Here's how the part is built. I have some questions about the finished solid (model axes, mm). Face numbers are marked on the shaded views. A direction names the side the tool comes from. Round coordinates to 2 decimals unless told otherwise and drop trailing zeros. Loops run counter-clockwise (first coordinate to the right, second up) from the corner with the lowest first, then second, coordinate; pieces in that order, holes last. Notation, with made-up numbers: (31.5, 59.5) -> (57.5, 59.5) arc R22 cw to (57.5, 72.5) -> close; hole circle Ø3 at (48.25, 22). An arc over 180 degrees is marked (long way). One line per item, written item: value. Start each with the question number.
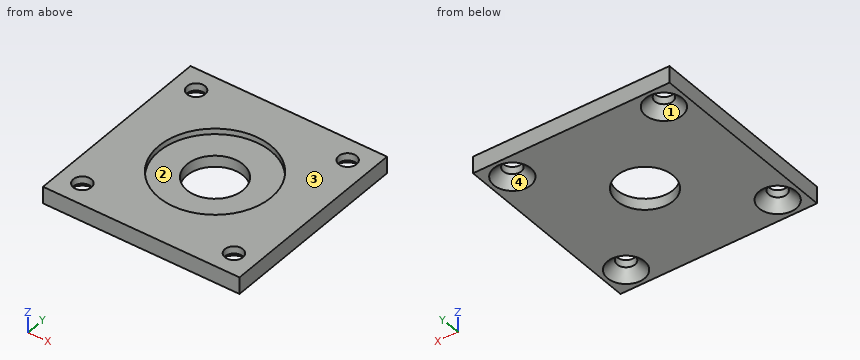
Autodesk Inventor part; units mm, degrees
ref_plane "YZ Plane" through (0, 0, 0) normal (1, 0, 0) x (0, 1, 0)
ref_plane "XZ Plane" through (0, 0, 0) normal (0, 1, 0) x (-1, 0, 0)
ref_plane "XY Plane" through (0, 0, 0) normal (0, 0, 1) x (1, 0, 0)
sketch "Sketch1" plane through (0, 0, 0) normal (0, 0, 1) x (1, 0, 0)
  line L0 (17.5, -17.5) -> (-17.5, -17.5)
  line L1 (-17.5, -17.5) -> (-17.5, 17.5)
  line L2 (-17.5, 17.5) -> (17.5, 17.5)
  line L3 (17.5, 17.5) -> (17.5, -17.5)
  line L4 (17.5, -17.5) -> (-17.5, 17.5) construction
  line L5 (-17.5, -17.5) -> (17.5, 17.5) construction
  circle A0 centre (-13.4987, -13.4987) radius 1.5
  circle A1 centre (13.4987, -13.4987) radius 1.5
  circle A2 centre (13.4987, 13.4987) radius 1.5
  circle A3 centre (-13.4987, 13.4987) radius 1.5
  circle A4 centre (0, 0) radius 5
  circle A5 centre (0, 0) radius 10
  dimension "d0" = 35
  dimension "d1" = 35
  dimension "d3" = 3
  dimension "d6" = 360
  dimension "d8" = 10
  dimension "d9" = 20
extrude "Extrusion1" add sketch "Sketch1" against normal blind 3 contours L0 L1 L2 L3 | A0 | A1 | A2 | A3 | A5
extrude "Extrusion2" cut sketch "Sketch1" against normal blind 1 contours A5
sketch "Sketch2" plane through (0, 0, -3) normal (0, 0, -1) x (-1, 0, 0)
  circle A0 centre (13.4987, 13.4987) radius 1.5
  circle A1 centre (-13.4987, 13.4987) radius 1.5
  circle A2 centre (-13.4987, -13.4987) radius 1.5
  circle A3 centre (13.4987, -13.4987) radius 1.5
  point P0 (0, 0)
hole "Hole2" at (13.4987, 13.4987, -3) at (-13.4987, 13.4987, -3) at (-13.4987, -13.4987, -3) at (13.4987, -13.4987, -3) direction (0, 0, 1) diameter 3.2 depth 3 countersink diameter 6.6 countersink angle 90
properties part number "АНЦП.014.00.00.004" material "PET Plastic"
Q1. Which directions (+Z, -Z, +X, -X, +Y, -Y) give clear straight access to the entire face, cutting with the end or side of a thin tool? Please do the marked faces 1 and 2.
Q2. If we mould it in two halves opening along Y, with no side actions, what happens to the marked faces 3 and 4? For each: released by +Y, released by -Y, zero draft, split by the parting line, or undercut.
Q3. If I drill on line 1 along Y through (x, z) = (-12, -1.9); line 2 along Y through (x, z) = (0, -2.15); line 3 along Y through (x, z) = (-13, -1.45), over which ranges is the centre line in solid material (lowest first)?
Q4. I want a section at D-D on x = -6. Please give me the cut outline in (y, z).
Q5. Will these pins go through, and if not, where does the flat tip stop? P1, Ø12, axis at x = 0, y = 0, coming from the +Z side; P2, Ø5, axis at x = 13.5, y = -13.5, coming from the -Z side.
Q6. I want a section at C-C on z = -0.5. Please give me the cut outline in (x, y).
Q7. I want a section at A-A on y = 0. Please give me the cut outline in (x, z), plus the area to 3 significant figures.
Answers below:
1. face 1: -Z
1. face 2: +Z
2. face 3: zero draft
2. face 4: undercut
3. line 1: y = -17.5 to -15.11, -11.89 to 11.89, 15.11 to 17.5
3. line 2: y = -17.5 to -5, 5 to 17.5
3. line 3: y = -17.5 to -15.18, -11.82 to 11.82, 15.18 to 17.5
4. outline: (-17.5, -3) -> (17.5, -3) -> (17.5, 0) -> (8, 0) -> (8, -1) -> (-8, -1) -> (-8, 0) -> (-17.5, 0) -> close
5. P1: stops at z = -1
5. P2: stops at z = -2.2
6. outline: (-17.5, -17.5) -> (17.5, -17.5) -> (17.5, 17.5) -> (-17.5, 17.5) -> close; hole circle Ø3.2 at (-13.5, -13.5); hole circle Ø3.2 at (-13.5, 13.5); hole circle Ø20 at (0, 0); hole circle Ø3.2 at (13.5, -13.5); hole circle Ø3.2 at (13.5, 13.5)
7. outline: (-17.5, -3) -> (-5, -3) -> (-5, -1) -> (-10, -1) -> (-10, 0) -> (-17.5, 0) -> close; (5, -3) -> (17.5, -3) -> (17.5, 0) -> (10, 0) -> (10, -1) -> (5, -1) -> close
7. area: 65.0 mm^2
